Could you check a few things on this drawing? It's one solid part, dimensions in mm from its lowest x, y, z. A direction names the side the tool comes from. Give positions to 0.01 mm unless a question says otherwise; leave off trailing zeros. Order: outer loops, then holes, each group sorted by start corner. A loop starts at its lowest first (then second) coordinate and runs counter-clockwise, first axis right, second up.
Item 1: Which directions (+Z, -Z, +X, -X, +Y, -Y) give clear straight access to the entire face, cutting with the end or side of a thin tool? Please do the marked faces 1, 2 and 3.
Item 2: I want a section at A-A, the plane z = 9. Write out the boundary of the cut face in (x, y), then the cut area to 3 significant figures.
Item 3: I want a section at C-C, the plane y = 4. Write out the boundary of the cut face in (x, z), then the cut area to 3 significant figures.
Item 4: If I drill on line 1 along Y through (x, z) = (9.75, 4.5); line 2 along Y through (x, z) = (1.75, 10); line 3 along Y through (x, z) = (10.25, 14.75), over which ranges is the centre line in solid material (lowest first)?
Item 5: If we mould it in two halves opening along Y, with no side actions, what happens to the marked faces 4, 5, 6 and 7? For each: +Y half, -Y half, draft (parallel to the pull), parting line (faces both ways), or undercut.
Item 6: I want a section at D-D, the plane y = 8.5. Write out the boundary of the cut face in (x, z), then the cut area to 3 significant figures.
Item 7: I'm going to push flat-ended pins straight in: pin 1 Ø6 at (x, y) = (12.5, 21) entering from -Z; pin 2 Ø8 at (x, y) = (4.5, 5) entering from -Z; pin 3 Ø5 at (y, z) = (11, 13) entering from -X. Where does each tip first touch, or does it pass through?
Item 8: I want a section at B-B, the plane x = 9. Write out the boundary of the cut face in (y, z).
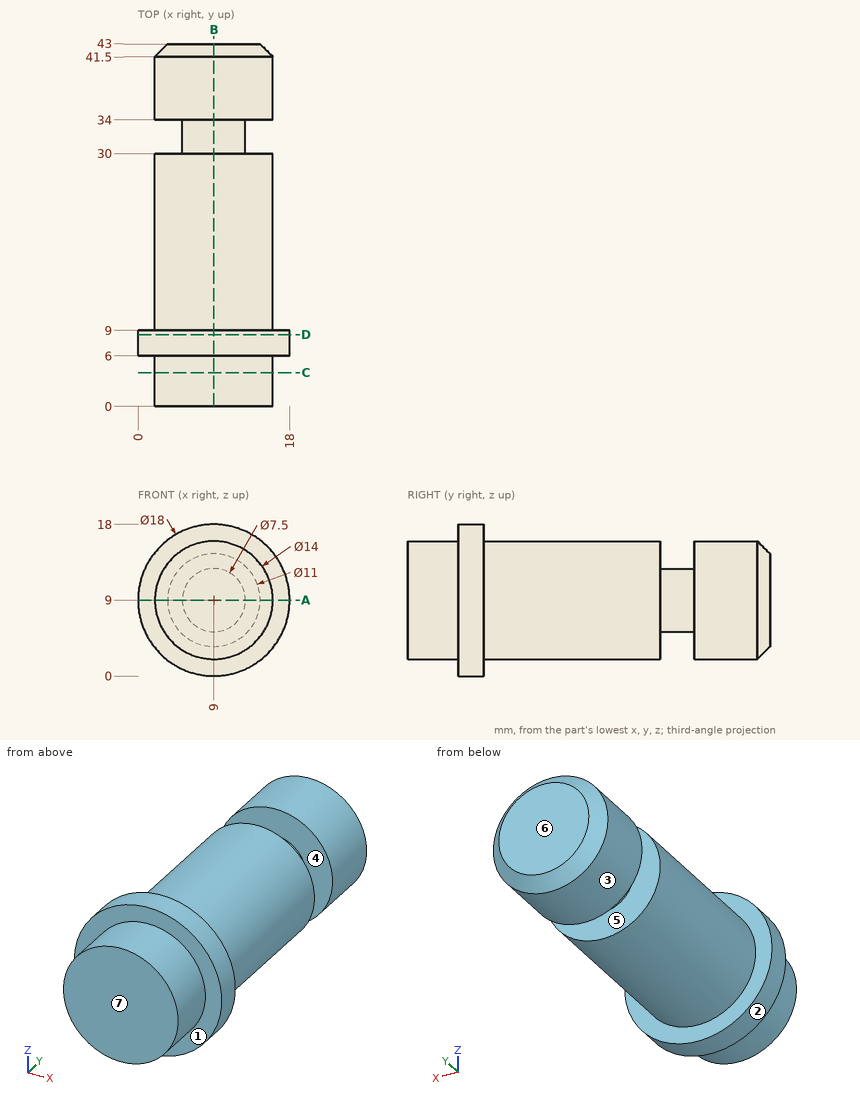
Results list:
1. face 1: -Y
1. face 2: +Y, -Y
1. face 3: +Y
2. outline: (0, 6) - (2, 6) - (2, 0) - (16, 0) - (16, 6) - (18, 6) - (18, 9) - (16, 9) - (16, 30) - (12.75, 30) - (12.75, 34) - (16, 34) - (16, 41.5) - (14.5, 43) - (3.5, 43) - (2, 41.5) - (2, 34) - (5.25, 34) - (5.25, 30) - (2, 30) - (2, 9) - (0, 9) - close
2. area: 586 mm2
3. outline: circle Ø14 at (9, 9)
3. area: 154 mm2
4. line 1: y = 0 to 30, 34 to 43
4. line 2: y = 6 to 9
4. line 3: y = 0 to 30, 34 to 42.62
5. face 4: undercut
5. face 5: undercut
5. face 6: +Y half
5. face 7: -Y half
6. outline: circle Ø18 at (9, 9)
6. area: 254 mm2
7. pin 1: stops at z = 2.02
7. pin 2: stops at z = 0.02
7. pin 3: stops at x = 0.35
8. outline: (0, 2) - (6, 2) - (6, 0) - (9, 0) - (9, 2) - (30, 2) - (30, 5.25) - (34, 5.25) - (34, 2) - (41.5, 2) - (43, 3.5) - (43, 14.5) - (41.5, 16) - (34, 16) - (34, 12.75) - (30, 12.75) - (30, 16) - (9, 16) - (9, 18) - (6, 18) - (6, 16) - (0, 16) - close
